Input: part model. Units: mm. Frame: model coordinates. Give positions to 0.01 mm unless a question says otherwise; leave off trailing zeros. Loops run counter-clockwise (first coordinate to the right, second up) from the corner with the lowest first, then second, coordinate; pieces in that order, holes last. Notation, with made-up numbers: (72, 22.25) - (110, 22.25) arc R9 cw to (110, 33.25) - close; hole circle Ø10 at (84.5, 27). An arc over 180 degrees is marked (long way). One line per item, written item: value.
from build123d import *

# Parameters (mm, degrees)
F0_R     = 2.5
F0_R_2   = 5
F1_DEPTH = 5


with BuildPart() as f1:
    # F0 (on Front) → F1 (new body)
    with BuildSketch(Plane.XZ):
        with BuildLine():
            Line((135.28383, -68.32226), (135.28383, -198.32226))
            Line((135.28383, -198.32226), (157.312748, -198.32226))
            Line((157.312748, -198.32226), (157.312748, -128.921397))
            ThreePointArc((157.312748, -128.921397), (152.769318, -123.942286), (157.312748, -118.963175))
            Line((157.312748, -118.963175), (157.312748, -105.930082))
            ThreePointArc((157.312748, -105.930082), (152.661874, -100.942286), (157.312748, -95.95449))
            Line((157.312748, -95.95449), (157.312748, -68.32226))
            Line((157.312748, -68.32226), (135.28383, -68.32226))
        make_face()
        with Locations((145.284414, -186.214134)):
            Circle(F0_R, mode=Mode.SUBTRACT)
        with Locations((145.284414, -178.556204)):
            Circle(F0_R, mode=Mode.SUBTRACT)
        with Locations((146.29881, -111.676522)):
            Circle(F0_R_2, mode=Mode.SUBTRACT)
        with BuildLine():
            Line((157.312748, -128.921397), (157.312748, -198.32226))
            Line((157.312748, -198.32226), (171.252168, -198.32226))
            ThreePointArc((171.252168, -198.32226), (177.252168, -196.336497), (180.882853, -191.163356))
            Line((180.882853, -191.163356), (179.799825, -75.244784))
            ThreePointArc((179.799825, -75.244784), (176.556179, -70.511493), (171.252168, -68.32226))
            Line((171.252168, -68.32226), (157.312748, -68.32226))
            Line((157.312748, -68.32226), (157.312748, -95.95449))
            ThreePointArc((157.312748, -95.95449), (161.07174, -97.2854), (162.661874, -100.942286))
            ThreePointArc((162.661874, -100.942286), (161.07174, -104.599172), (157.312748, -105.930082))
            Line((157.312748, -105.930082), (157.312748, -118.963175))
            ThreePointArc((157.312748, -118.963175), (161.139567, -120.248856), (162.769318, -123.942286))
            ThreePointArc((162.769318, -123.942286), (161.139567, -127.635716), (157.312748, -128.921397))
        make_face()
        with Locations((169.29881, -111.676522)):
            Circle(F0_R_2, mode=Mode.SUBTRACT)
    extrude(amount=F1_DEPTH)


solid = f1.part
Item 1: Section C-C, the plane y = -1.1. Output: boundary loops of the cut face in (x, z), and give its area (3 significant figures).
Verdict:
outline: (135.28, -198.32) - (171.25, -198.32) arc R10.06 ccw to (180.88, -191.16) - (179.8, -75.24) arc R10.06 ccw to (171.25, -68.32) - (135.28, -68.32) - close; hole circle Ø10 at (146.3, -111.68); hole circle Ø5 at (145.28, -186.21); hole circle Ø5 at (145.28, -178.56); hole circle Ø10 at (157.66, -100.94); hole (157.31, -128.92) arc R5 ccw to (162.77, -123.94) arc R5 ccw (long way) to start; hole circle Ø10 at (169.3, -111.68)
area: 5,470 mm^2
Item 2: Section D-D, the plane x = 146.5. Output: boundary loops of the cut face in (y, z), and give its area (3 significant figures).
Verdict:
outline: (-5, -198.32) - (0, -198.32) - (0, -188.4) - (-5, -188.4) - close; (-5, -184.03) - (0, -184.03) - (0, -180.74) - (-5, -180.74) - close; (-5, -176.37) - (0, -176.37) - (0, -116.67) - (-5, -116.67) - close; (-5, -106.68) - (0, -106.68) - (0, -68.32) - (-5, -68.32) - close
area: 556 mm^2
Item 3: Material intervals for L1, parallel to Z at x = 162, y = -0.65; L2, parallel to Z at x = 158.5, y = -3.95; L3, parallel to Z at x = 147.5, y = -3.7, sorted ascending.
Verdict:
L1: z = -198.32 to -126.61, -121.28 to -103.43, -98.46 to -68.32
L2: z = -198.32 to -128.89, -119 to -105.87, -96.01 to -68.32
L3: z = -198.32 to -187.37, -185.06 to -179.71, -177.4 to -116.53, -106.82 to -68.32
Item 4: Section B-B, the plane z = -103.5. Output: boundary loops of the cut face in (x, y).
Verdict:
outline: (135.28, -5) - (153.37, -5) - (153.37, 0) - (135.28, 0) - close; (161.96, -5) - (180.06, -5) - (180.06, 0) - (161.96, 0) - close
Item 5: Pin query (flat end, axial travel): P1, Ø8, axis at x = 169.3, z = -111.68, coming from the -Y side; P2, Ø6, axis at x = 145.28, z = -186.21, coming from the +Y side. Return the tip coordinate at first contact, or that it passes through.
Verdict:
P1: passes through
P2: stops at y = 0
Item 6: Section A-A, the plane x = 156. Output: boundary loops of the cut face in (y, z).
Verdict:
outline: (-5, -198.32) - (0, -198.32) - (0, -128.62) - (-5, -128.62) - close; (-5, -119.27) - (0, -119.27) - (0, -105.66) - (-5, -105.66) - close; (-5, -96.23) - (0, -96.23) - (0, -68.32) - (-5, -68.32) - close
Item 7: Draft query along X for faces 1 (the face through (158, -5, -132)), 2 (the face through (146.63, -2.46, -176.45)), 3 (the face through (135.284, -2, -132)), 4 (the face through (174.068, -2.465, -110.175)). Return one class per face: pulls with the +X half, pulls with the -X half, needs draft (parallel to the pull), parting line crosses it, or undercut.
Verdict:
face 1: needs draft
face 2: undercut
face 3: pulls with the -X half
face 4: undercut
